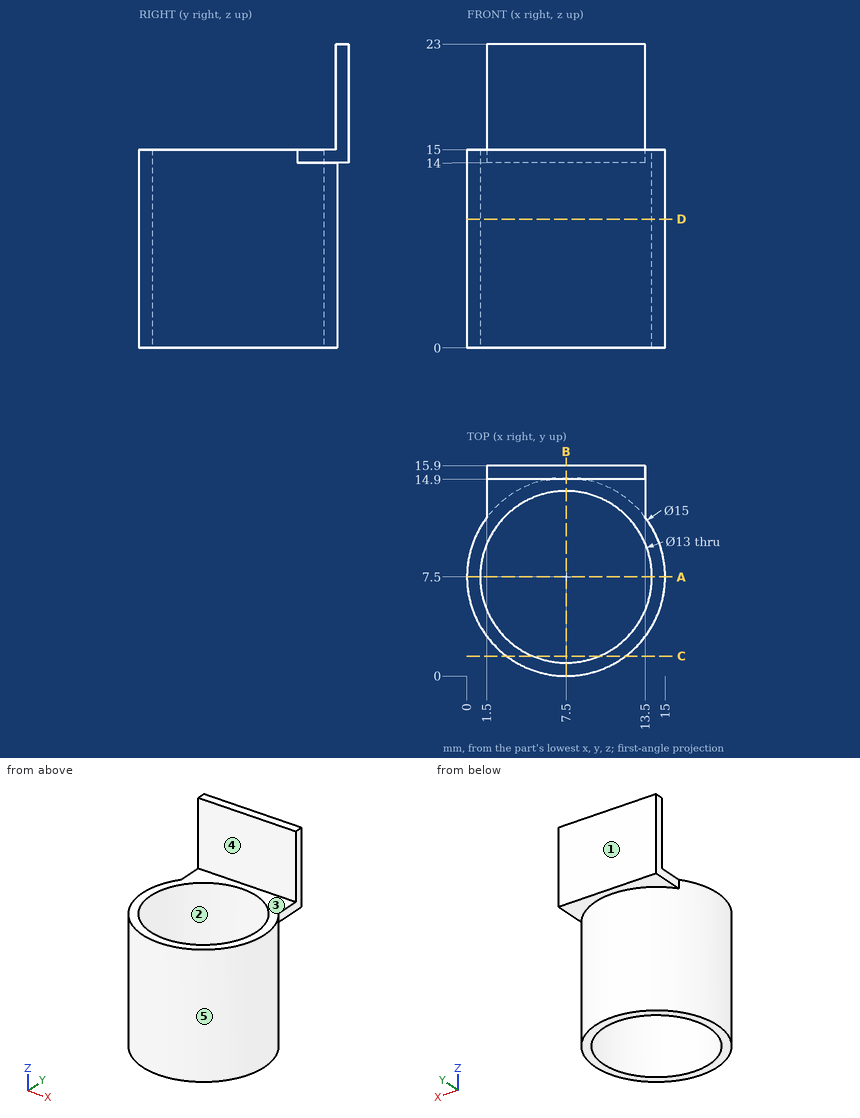
The drawing under review shows one solid part. Ordinate dimensions are in mm from its lowest x, y, z. A direction names the side the tool comes from. Coordinates: 2 decimals unless noted, no trailing zeros. Order: outer loops, then holes, each group sorted by start corner. A loop starts at its lowest first (then second) coordinate and runs counter-clockwise, first axis right, second up. Notation, with made-up numbers: (17.25, 61.25) -> (38.25, 61.25) arc R18 ccw to (38.25, 77.25) -> close; hole circle Ø5 at (-6.75, 38). An arc over 180 degrees is marked (long way). Return JSON: item names as keys, results as strings.
1. Machinability: for the marked faces 4 and 5, which of the approach directions +Z, -Z, +X, -X, +Y, -Y give a long, thin tool a straight path to every point of the face, cutting with its end or side? Answer none if there is none.
Answer block:
{"face 4": "+Z, +X, -X, -Y", "face 5": "-Z"}
2. The part is to be moulded in two halves that separate along Y. For the marked faces 1, 2 and 3, say which applies: +Y half, -Y half, draft (parallel to the pull), parting line (faces both ways), or undercut.
Answer block:
{"face 1": "+Y half", "face 2": "undercut", "face 3": "draft"}
3. We need section C-C on y = 1.5. Write out the cut boundary in (x, z), and give its area (3 significant figures).
Answer block:
{"outline": "(3, 0) -> (5, 0) -> (5, 15) -> (3, 15) -> close; (10, 0) -> (12, 0) -> (12, 15) -> (10, 15) -> close", "area": "60.0 mm²"}
4. We need section A-A on y = 7.5. Write out the cut boundary in (x, z), and give its area (3 significant figures).
Answer block:
{"outline": "(0, 0) -> (1, 0) -> (1, 15) -> (0, 15) -> close; (14, 0) -> (15, 0) -> (15, 15) -> (14, 15) -> close", "area": "30.0 mm²"}
5. For pin 1 Ø4.5 at (y, z) = (13.5, 20.5) entering from -X; pin 2 Ø1.5 at (x, y) = (2.5, 4) entering from +Z; pin 3 Ø2 at (x, z) = (5.5, 11.5) entering from -Y; pin 4 Ø2 at (y, z) = (4.5, 16.5) entering from -X, all flat-tipped, find the tip position at first contact; note any pin that passes through.
Answer block:
{"pin 1": "x = 1.5", "pin 2": "z = 15", "pin 3": "y = 0.07", "pin 4": "through"}
6. For line 1 (Y direction, x = 7.5, z = 7); line 2 (Y direction, x = 11, z = 15.25); line 3 (Z direction, x = 10.5, y = 14.75), list the stretches that pass through material, from the lowest coordinate up. Write a range as from..to.
Answer block:
{"line 1": "0..1, 14..15", "line 2": "14.9..15.9", "line 3": "14..15"}
7. We need section B-B on x = 7.5. Write out the cut boundary in (y, z), and give its area (3 significant figures).
Answer block:
{"outline": "(0, 0) -> (1, 0) -> (1, 15) -> (0, 15) -> close; (14, 0) -> (15, 0) -> (15, 14) -> (15.9, 14) -> (15.9, 23) -> (14.9, 23) -> (14.9, 15) -> (14, 15) -> close", "area": "38.9 mm²"}
8. We need section D-D on z = 9.75. Write out the cut boundary in (x, y).
Answer block:
{"outline": "circle Ø15 at (7.5, 7.5); hole circle Ø13 at (7.5, 7.5)"}
